```python
from build123d import *

# Parameters (mm, degrees)
F0_W     = 89
F0_H     = 45
F1_DEPTH = 5
F2_W     = 70
F2_H     = 39
F3_DEPTH = 25
F4_W     = 85.5
F4_H     = 41.5
F5_DEPTH = 3
F6_W     = 8
F6_H     = 8
F7_DEPTH = 3
F8_R     = 1.25
F8_R_2   = 1
F9_DEPTH = 25


with BuildPart() as f1:
    # F0 (on Top) → F1 (new body)
    with BuildSketch(Plane.XY):
        Rectangle(F0_W, F0_H)
    extrude(amount=F1_DEPTH)

    # F2 (on Top) → F3 (cut)
    with BuildSketch(Plane.XY):
        Rectangle(F2_W, F2_H)
    extrude(amount=F3_DEPTH, mode=Mode.SUBTRACT)

    # F4 (on Top) → F5 (cut)
    with BuildSketch(Plane.XY):
        Rectangle(F4_W, F4_H)
    extrude(amount=F5_DEPTH, mode=Mode.SUBTRACT)

    # F6 (on Top) → F7 (join)
    with BuildSketch(Plane.XY):
        with Locations((-40.5, 18.5)):
            Rectangle(F6_W, F6_H)
        with Locations((-40.5, -18.5)):
            Rectangle(F6_W, F6_H)
        with Locations((40.5, 18.5)):
            Rectangle(F6_W, F6_H)
        with Locations((40.5, -18.5)):
            Rectangle(F6_W, F6_H)
    extrude(amount=F7_DEPTH)

    # F8 (on Top) → F9 (cut)
    with BuildSketch(Plane.XY):
        with Locations((40.5, -18.5)):
            Circle(F8_R)
        with Locations((40.5, 18.5)):
            Circle(F8_R)
        with Locations((-40.5, -18.5)):
            Circle(F8_R)
        with Locations((-40.5, 18.5)):
            Circle(F8_R)
        with Locations((-39, 0)):
            Circle(F8_R_2)
        with Locations((39, 0)):
            Circle(F8_R_2)
    extrude(amount=F9_DEPTH, mode=Mode.SUBTRACT)


solid = f1.part
```
Geometry: final body of the model. Coordinates: model frame, mm. A direction names the side the tool comes from. Coordinates: 2 decimals unless noted, no trailing zeros. Write each loop counter-clockwise with the first axis right and the second up, starting at its lowest first coordinate (ties: lowest second). Pieces come first, ordered by that corner, then holes. Notation, with made-up numbers: M 82,18 L 103,18 A18 ccw 103,22 Z; hole C -13,55.5 d1. An arc over 180 degrees is marked long. Answer as CSV lines item,"result". Start each with the question number.
Q1. Reachability of faces 4 (the cylindrical face through (39.25, -18.45, 2.46)), 5 (the flat face through (40, 14.5, 1)) from +Z, -Z, +X, -X, +Y, -Y: full face, straight path, thin tool, end or side. Return the list, or none.
Q2. Cut plane A-A on x = -21.5. Return the cut outline in (y, z).
Q3. Cut plane B-B on y = -18.5. Return the cut outline in (x, z).
Q4. Line query: line 1 (X direction, y = -18.5, z = 2.65); line 2 (Y direction, x = 40.5, z = 3.95); line 3 (Y direction, x = 40.5, z = 2.8). Output: solid intervals per line, ascending. Write a range as from..to.
Q5. Mould query, pull axis X, two halves, no side actions, for faces 1 (the flat face through (44.5, 0, 2)), 2 (the flat face through (-1, -22.5, 2)), 3 (the flat face through (-1, -20.75, 1)). Classes: released by +X, released by -X, zero draft, split by the parting line, or undercut.
Q6. Cut plane C-C on z = 4.2. Return the cut outline in (x, y).
Q7. Cut plane D-D on y = -7.5. Return the cut outline in (x, z), then the cut area to 3 significant figures.
Findings below:
1,face 4,"+Z, -Z"
1,face 5,"-Z"
2,outline,"M -22.5,0 L -20.75,0 L -20.75,3 L -19.5,3 L -19.5,5 L -22.5,5 Z; M 19.5,3 L 20.75,3 L 20.75,0 L 22.5,0 L 22.5,5 L 19.5,5 Z"
3,outline,"M -44.5,0 L -41.75,0 L -41.75,5 L -44.5,5 Z; M -39.25,0 L -36.5,0 L -36.5,3 L -35,3 L -35,5 L -39.25,5 Z; M 35,3 L 36.5,3 L 36.5,0 L 39.25,0 L 39.25,5 L 35,5 Z; M 41.75,0 L 44.5,0 L 44.5,5 L 41.75,5 Z"
4,line 1,"x = -44.5..-41.75, -39.25..-36.5, 36.5..39.25, 41.75..44.5"
4,line 2,"y = -22.5..-19.75, -17.25..17.25, 19.75..22.5"
4,line 3,"y = -22.5..-19.75, -17.25..-14.5, 14.5..17.25, 19.75..22.5"
5,face 1,"released by +X"
5,face 2,"zero draft"
5,face 3,"undercut"
6,outline,"M -44.5,-22.5 L 44.5,-22.5 L 44.5,22.5 L -44.5,22.5 Z; hole C -40.5,-18.5 d2.5; hole C -40.5,18.5 d2.5; hole C -39,0 d2; hole M -35,-19.5 L 35,-19.5 L 35,19.5 L -35,19.5 Z; hole C 39,0 d2; hole C 40.5,-18.5 d2.5; hole C 40.5,18.5 d2.5"
7,outline,"M -44.5,0 L -42.75,0 L -42.75,3 L -35,3 L -35,5 L -44.5,5 Z; M 35,3 L 42.75,3 L 42.75,0 L 44.5,0 L 44.5,5 L 35,5 Z"
7,area,"48.5 mm2"
